Drawing for the job (mm, zero at the part's lowest x, y, z). A direction names the side the tool comes from. Give positions to 0.01 mm unless a question says otherwise; leave off trailing zeros. Write each loop counter-clockwise with the first axis right and the second up, starting at its lowest first coordinate (ties: lowest second). Pieces come first, ordered by that corner, then holes.
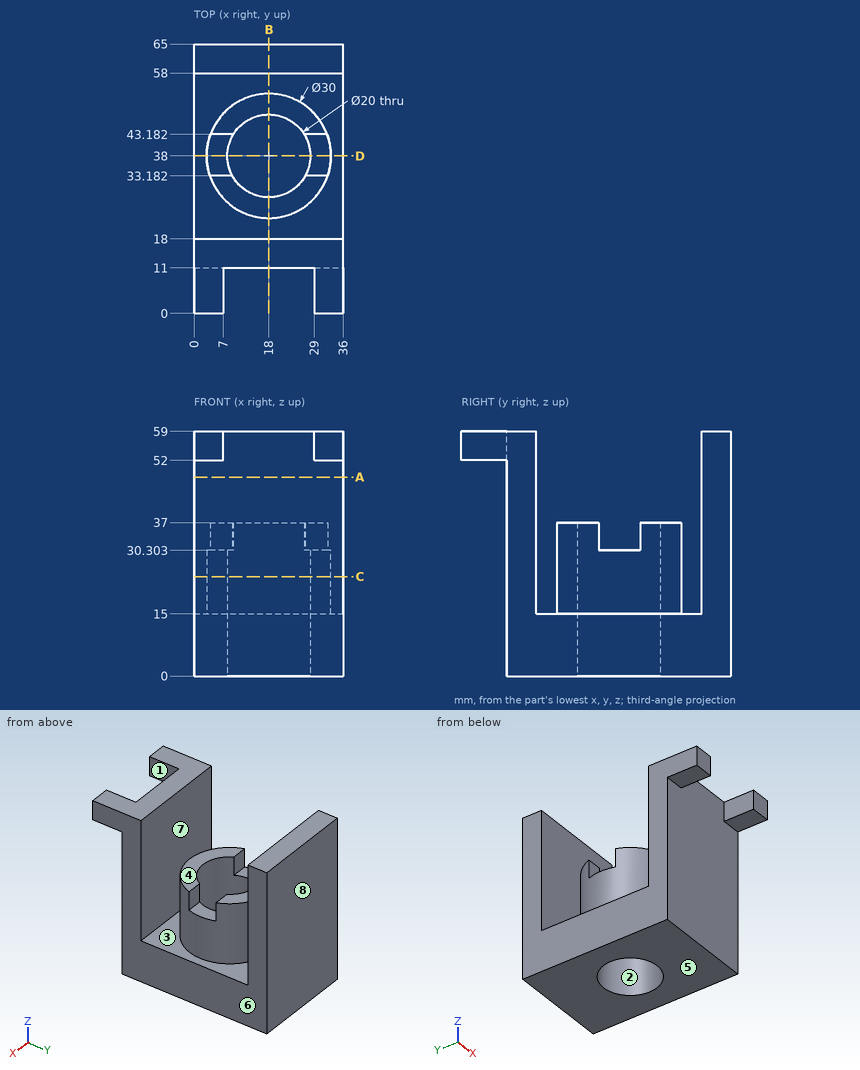
1. Probe probe 1 along Y at (x, z) = (18, 25); probe 2 along Y at (x, z) = (23, 55.5); probe 3 along Y at (x, z) = (11, 20.5) (1 decimal). List the from-to ranges inside material, lowest first.
Calculated:
probe 1: y = 11 to 18, 23 to 28, 48 to 53, 58 to 65
probe 2: y = 11 to 18, 58 to 65
probe 3: y = 11 to 18, 24.7 to 30.9, 45.1 to 51.3, 58 to 65
2. Slice it at A-A, the plane z = 48. Write the cut outline in (x, y).
Calculated:
outline: (0, 11) - (36, 11) - (36, 18) - (0, 18) - close; (0, 58) - (36, 58) - (36, 65) - (0, 65) - close
3. Slice it at C-C, the plane z = 24. Write the cut outline in (x, y).
Calculated:
outline: (0, 11) - (36, 11) - (36, 18) - (0, 18) - close; (0, 58) - (36, 58) - (36, 65) - (0, 65) - close; circle Ø30 at (18, 38); hole circle Ø20 at (18, 38)
4. Slice it at B-B, the plane x = 18. Write the cut outline in (y, z), and give its area (3 significant figures).
Calculated:
outline: (11, 0) - (28, 0) - (28, 37) - (23, 37) - (23, 15) - (18, 15) - (18, 59) - (11, 59) - close; (48, 0) - (65, 0) - (65, 59) - (58, 59) - (58, 15) - (53, 15) - (53, 37) - (48, 37) - close
area: 1,350 mm2
5. Pin check, flat tips, straight feed: P1, Ø8, axis at y = 23, z = 18.5, coming from the +X side; P2, Ø3, axis at x = 6, y = 36, coming from the +Z side; P3, Ø3, axis at x = 14.5, y = 29.5, coming from the +Z side; P4, Ø6, axis at x = 21.5, z = 48, coming from the -Y side. Stop position of each tip, or through.
Calculated:
P1: stops at x = 36
P2: stops at z = 30.3
P3: stops at z = 37
P4: stops at y = 11
6. Which spindle directions (+Z, -Z, +X, -X, +Y, -Y) get a long thin tool onto all of the face, cutting with end or side? Do the marked faces 1, 2, 3, 4 and 5. Say none if no direction does.
Calculated:
face 1: +Z, -Z, -Y
face 2: +Z, -Z
face 3: +Z
face 4: +Z, +X, -X
face 5: -Z, +X, -X, +Y, -Y
7. Slice it at D-D, the plane y = 38. Write the cut outline in (x, z).
Calculated:
outline: (0, 0) - (8, 0) - (8, 30.3) - (3, 30.3) - (3, 15) - (0, 15) - close; (28, 0) - (36, 0) - (36, 15) - (33, 15) - (33, 30.3) - (28, 30.3) - close
8. Pull direction Y, two halves, no side cores. Call the marked faces 6, 7 and 8: +Y half, -Y half, draft (parallel to the pull), parting line (faces both ways), or undercut.
Calculated:
face 6: draft
face 7: undercut
face 8: +Y half
